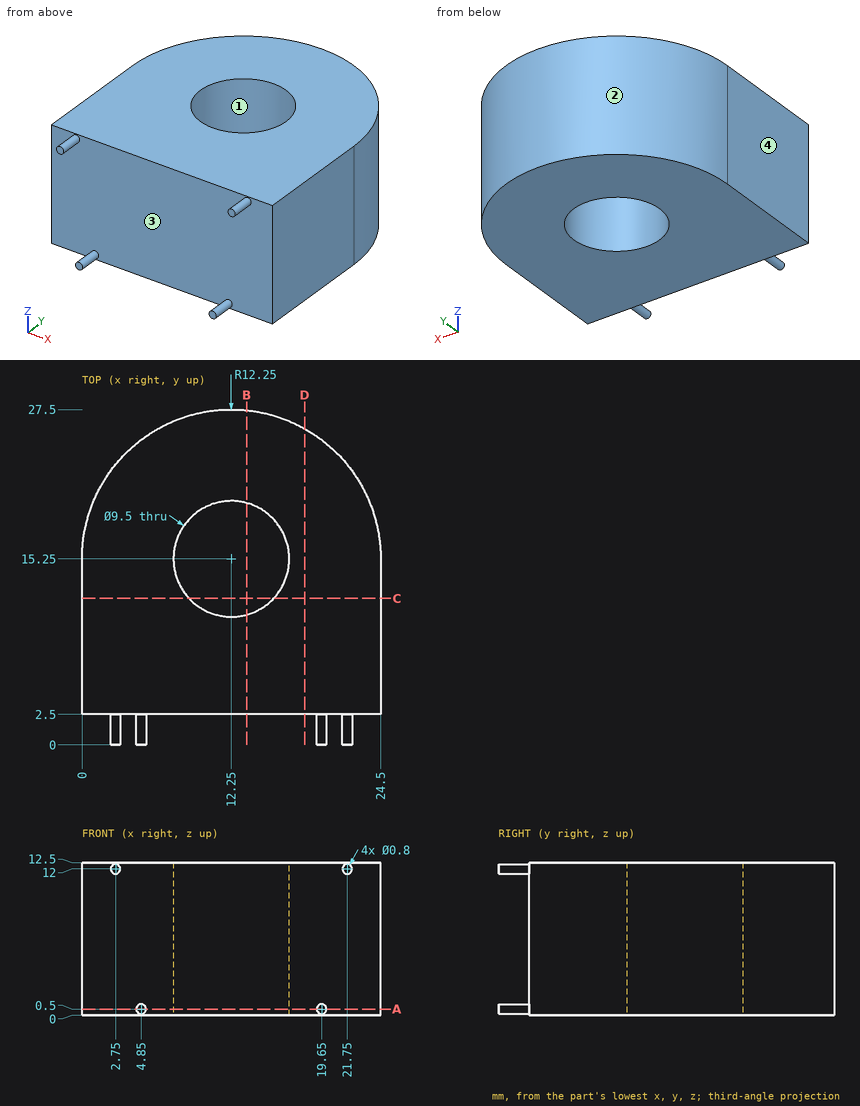
Geometry check sheet. Reference: drawing and pictorial views, mm from the part's lowest x, y, z. Give positions to 0.01 mm unless a question says otherwise; leave off trailing zeros. Loops run counter-clockwise (first coordinate to the right, second up) from the corner with the lowest first, then second, coordinate; pieces in that order, holes last. Notation, with made-up numbers: (-35, 17) -> (-21, 17) arc R29 ccw to (-21, 37) -> close; hole circle Ø7 at (23.25, 50.5). An arc over 180 degrees is marked (long way). Answer in a Markdown table with one row per item. Add a question column.
1) Cross-section at D-D on x = 18.25. Record the boundary of the cut face in (y, z).
2) Material ranges on probe 1 along Y at (x, z) = (12.25, 10); probe 2 along Y at (x, z) = (9.75, 4.75); probe 3 along X at (y, z) = (11, 12), recorded low to high. Write a range as from..to.
3) Gauge pin test, flat ends, axial feed: P1, Ø7.5, axis at x = 12.25, y = 15.25, coming from the +Z side; P2, Ø4, axis at x = 8, z = 7, coming from the -Y side. Record the tip position at first contact, or that the pin passes through.
4) Cross-section at C-C on y = 12. Record the boundary of the cut face in (x, z).
5) Cross-section at A-A on z = 0.5. Record the boundary of the cut face in (x, y).
6) Cross-section at B-B on x = 13.5. Record the boundary of the cut face in (y, z).
7) Draft check along Y on the marked faces 1, 2, 3 and 4. Enter one of: pulls with the +Y half, pulls with the -Y half, needs draft (parallel to the pull), parting line crosses it, or undercut.
Outcome:
| question | item | result |
|---|---|---|
| 1 | outline | (2.5, 0) -> (25.93, 0) -> (25.93, 12.5) -> (2.5, 12.5) -> close |
| 2 | probe 1 | y = 2.5..10.5, 20..27.5 |
| 2 | probe 2 | y = 2.5..11.21, 19.29..27.24 |
| 2 | probe 3 | x = 0..10.13, 14.37..24.5 |
| 3 | P1 | passes through |
| 3 | P2 | stops at y = 2.5 |
| 4 | outline | (0, 0) -> (8.79, 0) -> (8.79, 12.5) -> (0, 12.5) -> close; (15.71, 0) -> (24.5, 0) -> (24.5, 12.5) -> (15.71, 12.5) -> close |
| 5 | outline | (0, 2.5) -> (4.45, 2.5) -> (4.45, 0) -> (5.25, 0) -> (5.25, 2.5) -> (19.25, 2.5) -> (19.25, 0) -> (20.05, 0) -> (20.05, 2.5) -> (24.5, 2.5) -> (24.5, 15.25) arc R12.25 ccw to (0, 15.25) -> close; hole circle Ø9.5 at (12.25, 15.25) |
| 6 | outline | (2.5, 0) -> (10.67, 0) -> (10.67, 12.5) -> (2.5, 12.5) -> close; (19.83, 0) -> (27.44, 0) -> (27.44, 12.5) -> (19.83, 12.5) -> close |
| 7 | face 1 | undercut |
| 7 | face 2 | pulls with the +Y half |
| 7 | face 3 | pulls with the -Y half |
| 7 | face 4 | needs draft |
